Can you work these out from the model? Positions are in its coordinate system, mm. Give positions to 0.01 mm unless a question says otherwise; leave off trailing zeros. Order: outer loops, then holes, each group sorted by start corner. A loop starts at its lowest first (then second) coordinate and runs counter-clockwise, first axis right, second up. Notation, with made-up numbers: M 62.5,-32.75 L 101.5,-32.75 A12 cw 101.5,-26.75 Z; hole C 49.25,39.25 d7. An arc over 180 degrees is marked long. Use one line per item in the form item = value. Start each with the question number.
1. I want a section at A-A, the plane z = 3.5. List the corners of the cut face in (x, y) for me, and give its area (3 significant figures).
2. I need wall thicknesses on L1, parallel to Y at x = 40, z = 1.3; L2, parallel to Z at x = 18, y = -0.1; L3, parallel to X at y = -1.7, z = 8.25. Which ranges of each line are inside material? Lowest first, please.
3. I want a section at B-B, the plane x = 36. List the corners of the cut face in (y, z) for me.
4. Will these pins go through, and if not, where does the flat tip stop? P1, Ø2, axis at y = 1.5, z = 8.5, coming from the -X side; P2, Ø2, axis at y = -1, z = 8.5, coming from the +X side; P3, Ø1.5, axis at x = 10.5, y = -1, coming from the +Z side.
5. We'd pull the mould along Y, two halves only. Please class faces 1 (the face through (20, 2, 1)), 2 (the face through (40.715, 0.225, 1.014)), 3 (the face through (42, 0, 1)): +Y half, -Y half, draft (parallel to the pull), parting line (faces both ways), or undercut.
```python
from build123d import *

# Parameters (mm, degrees)
BOSS_EXTRUDE1_DEPTH   = 2
SKETCH2_R             = 2
BOSS_EXTRUDE2_DEPTH   = 8
CROQUIS1_R            = 0.75
CORTAR_EXTRUIR1_DEPTH = 10


with BuildPart() as part:
    # Sketch1 → Boss-Extrude1 (new body)
    with BuildSketch(Plane.XY):
        with BuildLine():
            Line((0, -2), (40, -2))
            ThreePointArc((40, -2), (42, 0), (40, 2))
            Line((40, 2), (0, 2))
            ThreePointArc((0, 2), (-2, 0), (0, -2))
        make_face()
    extrude(amount=BOSS_EXTRUDE1_DEPTH)

    # Sketch2 → Boss-Extrude2 (add)
    with BuildSketch(Plane.XY.offset(2)):
        with Locations(Location((0, 0, 0), (0, 0, 270))):
            Circle(SKETCH2_R)
    extrude(amount=BOSS_EXTRUDE2_DEPTH)

    # Croquis1 → Cortar-Extruir1 (cut)
    with BuildSketch(Plane.XY.offset(2)):
        with Locations((40, 0)):
            Circle(CROQUIS1_R)
    extrude(amount=-CORTAR_EXTRUIR1_DEPTH, mode=Mode.SUBTRACT)


solid = part.part
```
Check result:
q1.outline = C 0,0 d4
q1.area = 12.6 mm2
q2.L1 = -2 to -0.75, 0.75 to 2
q2.L2 = 0 to 2
q2.L3 = -1.05 to 1.05
q3.outline = M -2,0 L 2,0 L 2,2 L -2,2 Z
q4.P1 = -1.94
q4.P2 = 2
q4.P3 = 2
q5.face_1 = +Y half
q5.face_2 = undercut
q5.face_3 = parting line
